Work out the finished part from the listing and answer in its coordinate system (mm). Round coordinates to 2 decimals unless told otherwise and drop trailing zeros. Order: outer loops, then holes, each group sorted by start corner. A loop starts at its lowest first (then second) coordinate and runs counter-clockwise, first axis right, second up. Notation, with made-up numbers: (48, 47) - (97, 47) arc R26 cw to (97, 84) - close; hole circle Ø4 at (-10, 78.25). An arc over 180 degrees is marked (long way). Answer in a Markdown table with one row per item.
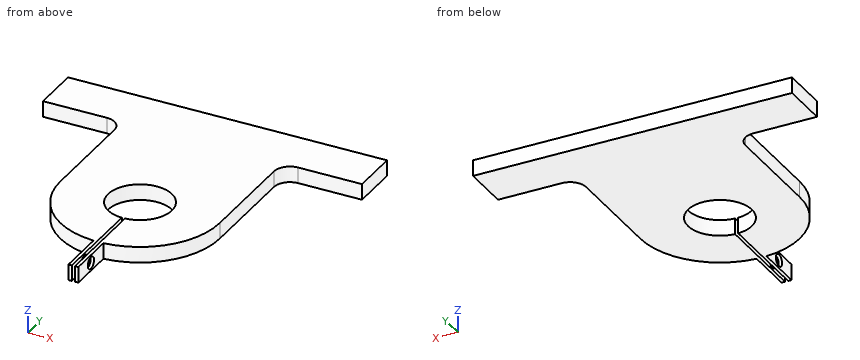
from build123d import *

# Parameters (mm, degrees)
BOSS_EXTRUDE1_DEPTH = 5.08
SKETCH4_R           = 1.905
CUT_EXTRUDE2_DEPTH  = 75.926658634


with BuildPart() as part:
    # Sketch1 → Boss-Extrude1 (new body)
    with BuildSketch(Plane.XY):
        with BuildLine():
            Line((-25.4, 0), (-25.4, 33.02))
            ThreePointArc((-25.4, 33.02), (-26.887897552, 36.612102448), (-30.48, 38.1))
            Line((-30.48, 38.1), (-50.8, 38.1))
            Line((-50.8, 38.1), (-50.8, 53.34))
            Line((-50.8, 53.34), (50.8, 53.34))
            Line((50.8, 53.34), (50.8, 38.1))
            Line((50.8, 38.1), (30.48, 38.1))
            ThreePointArc((30.48, 38.1), (26.887897552, 36.612102448), (25.4, 33.02))
            Line((25.4, 33.02), (25.4, 0))
            ThreePointArc((25.4, 0), (18.508661853, -17.395098057), (1.574060126, -25.351180145))
            Line((1.574060126, -25.351180145), (1.574060126, -40.634919492))
            Line((1.574060126, -40.634919492), (0.508, -40.634919492))
            Line((0.508, -40.634919492), (0.508, -25.394919492))
            Line((0.508, -25.394919492), (0.508, -10.147292053))
            ThreePointArc((0.508, -10.147292053), (0, 10.16), (-0.508, -10.147292053))
            Line((-0.508, -10.147292053), (-0.508, -25.394919492))
            Line((-0.508, -25.394919492), (-0.508, -40.634919492))
            Line((-0.508, -40.634919492), (-1.574060126, -40.634919492))
            Line((-1.574060126, -40.634919492), (-1.574060126, -25.351180145))
            ThreePointArc((-1.574060126, -25.351180145), (-18.508661853, -17.395098057), (-25.4, 0))
        make_face()
    extrude(amount=BOSS_EXTRUDE1_DEPTH)

    # Sketch4 → Cut-Extrude2 (cut, through all)
    with BuildSketch(Plane(origin=(1.574060126, 0, 0), x_dir=(0, 0, -1), z_dir=(1, 0, 0))):
        with Locations(Location((-2.54, -32.971180145, 0), (0, 0, 90))):
            Circle(SKETCH4_R)
    extrude(amount=-CUT_EXTRUDE2_DEPTH, mode=Mode.SUBTRACT)


solid = part.part
1) Find section D-D, the plane y = 19. Give the vertices of the cut face in (x, z), then the cut area to 3 significant figures.
Filled in:
| item | result |
|---|---|
| outline | (-25.4, 0) - (25.4, 0) - (25.4, 5.08) - (-25.4, 5.08) - close |
| area | 258 mm^2 |
2) Find section C-C, the plane x = 5.5. Give the vertices of the cut face in (y, z), then the cut area to 3 significant figures.
Filled in:
| item | result |
|---|---|
| outline | (-24.8, 0) - (-8.54, 0) - (-8.54, 5.08) - (-24.8, 5.08) - close; (8.54, 0) - (53.34, 0) - (53.34, 5.08) - (8.54, 5.08) - close |
| area | 310 mm^2 |
3) Find section A-A, the plane z = 2.54. Give the vertices of the cut face in (x, y).
Filled in:
| item | result |
|---|---|
| outline | (-50.8, 38.1) - (-30.48, 38.1) arc R5.08 cw to (-25.4, 33.02) - (-25.4, 0) arc R25.4 ccw to (-1.57, -25.35) - (-1.57, -31.07) - (-0.51, -31.07) - (-0.51, -10.15) arc R10.16 cw (long way) to (0.51, -10.15) - (0.51, -31.07) - (1.57, -31.07) - (1.57, -25.35) arc R25.4 ccw to (25.4, 0) - (25.4, 33.02) arc R5.08 cw to (30.48, 38.1) - (50.8, 38.1) - (50.8, 53.34) - (-50.8, 53.34) - close; (-1.57, -40.63) - (-0.51, -40.63) - (-0.51, -34.88) - (-1.57, -34.88) - close; (0.51, -40.63) - (1.57, -40.63) - (1.57, -34.88) - (0.51, -34.88) - close |
4) Find the intervals of material crossed by probe 1 along X at (y, z) = (-36, 1.1); probe 2 along X at (y, z) = (-11, 0.3); probe 3 along X at (y, z) = (32, 1.15), in increasing order. Write a range as from..to.
Filled in:
| item | result |
|---|---|
| probe 1 | x = -1.57..-0.51, 0.51..1.57 |
| probe 2 | x = -22.89..-0.51, 0.51..22.89 |
| probe 3 | x = -25.4..25.4 |
5) Each of these flat-tipped pins is pushed along its axis until it touches: pin 1 (1.5 mm diameter, centred on y = -33, z = 2, fed in from +X); pin 2 (1.5 mm diameter, centred on x = 38, z = 3, fed in from -Y); pin 3 (1 mm diameter, centred on y = -22, z = 3, fed in from +X); pin 4 (2 mm diameter, centred on x = 27, y = 39, fed in from -Z). Where does it stop, or does it pass through?
Filled in:
| item | result |
|---|---|
| pin 1 | passes through |
| pin 2 | stops at y = 38.1 |
| pin 3 | stops at x = 13.52 |
| pin 4 | stops at z = 0 |
6) Find section B-B, the plane y = -23.5. Give the vertices of the cut face in (x, z).
Filled in:
| item | result |
|---|---|
| outline | (-9.64, 0) - (-0.51, 0) - (-0.51, 5.08) - (-9.64, 5.08) - close; (0.51, 0) - (9.64, 0) - (9.64, 5.08) - (0.51, 5.08) - close |
